The listing builds one solid part. Answer for the finished solid, in the listing's coordinates (mm). Face numbers are marked on the shaded views. A direction names the side the tool comes from. Round coordinates to 2 decimals unless told otherwise and drop trailing zeros. Write each loop counter-clockwise with the first axis right and the second up, starting at its lowest first coordinate (ties: lowest second). Pieces come first, ordered by that corner, then holes. Notation, with made-up numbers: (9.25, 21) - (62.25, 21) arc R20 cw to (62.25, 59) - close; hole circle Ø8 at (44.25, 1.5). An arc over 180 degrees is marked (long way). Return JSON: item names as keys, results as strings. Group by question number.
(1) Find the intervals of material crossed by line 1 along Y through (x, z) = (-3.5, -11.5); line 2 along Y through (x, z) = (1, 17.5); line 3 along Z through (x, y) = (-11, 293), in increasing order. Write a range as [from, to].
(2) Section A-A, the plane y = 326 is taken. Write down the section's boundary in (x, z).
(3) Determine the mould class of the marked faces 3, 4 and 5 for opening direction Y: +Y half, -Y half, draft (parallel to the pull), parting line (faces both ways), or undercut.
(4) Each of these flat-tipped pins is pushed along its axis until it touches: pin 1 (2 mm diameter, centred on y = 87, z = -5, fed in from -X); pin 2 (2 mm diameter, centred on x = -8.5, y = 338.5, fed in from +Z); pin 3 (4 mm diameter, centred on x = 1.5, y = 0.5, fed in from -Z); pin 4 (8.5 mm diameter, centred on x = 5.5, y = 208, fed in from -Z). Where does it stop, or does it pass through?
(5) Which of the six approach directions +Z, -Z, +X, -X, +Y, -Y give full straight-line access (tool end or side, diameter ignored) to the marked faces 1 and 2?
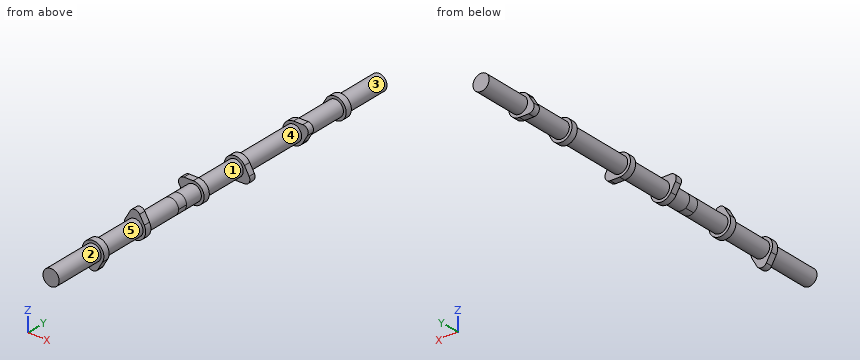
```python
from build123d import *

# Parameters (mm, degrees)
BOSS_EXTRUDE1_DEPTH      = 3.81
BODY_MOVE_COPY2_ANGLE    = 180
BOSS_EXTRUDE2_START      = -25.4
SKETCH2_R                = 9.5
BOSS_EXTRUDE2_DEPTH      = 146.05
BOSS_EXTRUDE2_DEPTH_BACK = 11.7
LPATTERN1_COUNT          = 3
LPATTERN1_PITCH          = 146.05
BODY_MOVE_COPY3_ANGLE    = 120
BODY_MOVE_COPY4_ANGLE    = 120
SKETCH3_R                = 9.5
BOSS_EXTRUDE3_DEPTH      = 27.94


with BuildPart() as part:
    # Sketch1 → Boss-Extrude1 (new body, symmetric)
    with BuildSketch(Plane(origin=(0, 0, 0), x_dir=(1, 0, 0), z_dir=(0, 1, 0))):
        with BuildLine():
            Line((-5.499261314, 15.875), (-10.998522628, 6.35))
            ThreePointArc((-10.998522628, 6.35), (0, -12.7), (10.998522628, 6.35))
            Line((10.998522628, 6.35), (5.499261314, 15.875))
            ThreePointArc((5.499261314, 15.875), (0, 19.05), (-5.499261314, 15.875))
        make_face()
    extrude(amount=BOSS_EXTRUDE1_DEPTH, both=True)


with BuildPart() as body_2:
    # Body-Move_Copy1: copy of part
    add(part.part.moved(Location((0, 60.96, 0))))


with BuildPart() as body_2_1:
    # Body-Move_Copy2: moved
    add(body_2.part.rotate(Axis((0, 0, 0), (0, 1, 0)), BODY_MOVE_COPY2_ANGLE))


with BuildPart() as part_1:
    add(part.part)

    add(body_2_1.part)  # Boss-Extrude2 merges body 2
    # Sketch2 → Boss-Extrude2 (add, two sides)
    with BuildSketch(Plane(origin=(0, 0, 0), x_dir=(1, 0, 0), z_dir=(0, 1, 0)).offset(BOSS_EXTRUDE2_START)) as boss_extrude2_sk:
        Circle(SKETCH2_R)
    extrude(amount=BOSS_EXTRUDE2_DEPTH)
    extrude(boss_extrude2_sk.sketch, amount=-BOSS_EXTRUDE2_DEPTH_BACK)


with BuildPart() as lpattern1_1:
    # LPattern1: pattern copy
    add(part_1.part.moved(Location(Vector(0, 1, 0) * (1 * LPATTERN1_PITCH))))


with BuildPart() as lpattern1_2:
    # LPattern1: pattern copy
    add(part_1.part.moved(Location(Vector(0, 1, 0) * (2 * LPATTERN1_PITCH))))


with BuildPart() as lpattern1_1_1:
    # Body-Move_Copy3: moved
    add(lpattern1_1.part.rotate(Axis((0, 0, 0), (0, 1, 0)), BODY_MOVE_COPY3_ANGLE))


with BuildPart() as lpattern1_2_1:
    # Body-Move_Copy4: moved
    add(lpattern1_2.part.rotate(Axis((0, 0, 0), (0, -1, 0)), BODY_MOVE_COPY4_ANGLE))


with BuildPart() as lpattern1_1_2:
    add(lpattern1_1_1.part)

    # Combine1: union LPattern1_2, part
    add(lpattern1_2_1.part)
    add(part_1.part)

    # Sketch3 → Boss-Extrude3 (add)
    with BuildSketch(Plane.XZ.offset(37.1)):
        Circle(SKETCH3_R)
    extrude(amount=BOSS_EXTRUDE3_DEPTH)


solid = lpattern1_1_2.part
```
Working result:
{
 "1": {"line 1": "y = [-3.81, 3.81], [57.15, 64.77], [142.24, 149.86], [203.2, 210.82], [288.29, 295.91], [349.25, 356.87]", "line 2": "y = [57.15, 64.77]", "line 3": "z = [-6.35, 6.35]"},
 "2": {"outline": "circle Ø19 at (0, 0)"},
 "3": {"face 3": "draft", "face 4": "undercut", "face 5": "undercut"},
 "4": {"pin 1": "stops at x = -8.62", "pin 2": "stops at z = 5.83", "pin 3": "stops at z = -19.05", "pin 4": "stops at z = -12.7"},
 "5": {"face 1": "none", "face 2": "-Y"}
}
